Print and shaded views of the part. All mm, measured from the part's lowest x, y and z. A direction names the side the tool comes from. Round coordinates to 2 decimals unless told otherwise and drop trailing zeros. Order: outer loops, then holes, each group sorted by start corner. A loop starts at its lowest first (then second) coordinate and runs counter-clockwise, first axis right, second up. Notation, with made-up numbers: (-15.5, 61.25) -> (19.5, 61.25) arc R21 ccw to (19.5, 93.25) -> close; hole circle Ø5 at (3.25, 69). An arc over 180 degrees is marked (long way). Answer as CSV lines item,"result".
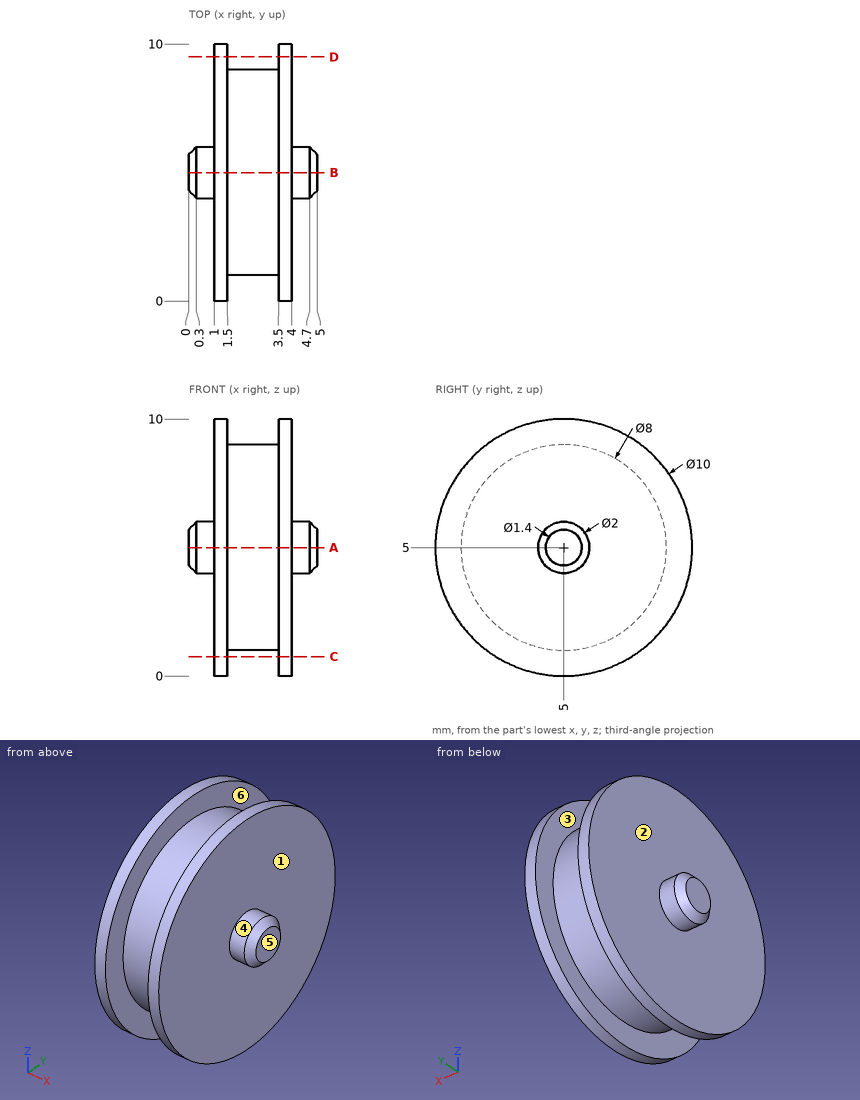
Q1. Saw through at A-A (z = 5). Write the cut outline in (x, y), plus the area to 3 significant figures.
Checks:
outline,"(0, 4.3) -> (0.3, 4) -> (1, 4) -> (1, 0) -> (1.5, 0) -> (1.5, 1) -> (3.5, 1) -> (3.5, 0) -> (4, 0) -> (4, 4) -> (4.7, 4) -> (5, 4.3) -> (5, 5.7) -> (4.7, 6) -> (4, 6) -> (4, 10) -> (3.5, 10) -> (3.5, 9) -> (1.5, 9) -> (1.5, 10) -> (1, 10) -> (1, 6) -> (0.3, 6) -> (0, 5.7) -> close"
area,"29.8 mm²"
Q2. Flat gauge pin, fed straight in: pin 1 (3 mm diameter, centred on y = 2.5, z = 5.5, fed in from +X). Where does the tip first touch, or does it go through?
Checks:
pin 1,"x = 4"
Q3. Saw through at D-D (y = 9.5). Write the cut outline in (x, z).
Checks:
outline,"(1, 2.82) -> (1.5, 2.82) -> (1.5, 7.18) -> (1, 7.18) -> close; (3.5, 2.82) -> (4, 2.82) -> (4, 7.18) -> (3.5, 7.18) -> close"
Q4. Mould opens along X. For the marked faces 1, 2, 3 and 4 say: +X half, -X half, draft (parallel to the pull), parting line (faces both ways), or undercut.
Checks:
face 1,"+X half"
face 2,"-X half"
face 3,"undercut"
face 4,"draft"
Q5. Tool access for the marked faces 5 and 6: list every direction of +Z, -Z, +X, -X, +Y, -Y with a clear straight run to the whole face (end or side of a thin tool).
Checks:
face 5,"+Z, -Z, +X, +Y, -Y"
face 6,"none"
Q6. Saw through at C-C (z = 0.75). Write the cut outline in (x, y).
Checks:
outline,"(1, 2.37) -> (1.5, 2.37) -> (1.5, 7.63) -> (1, 7.63) -> close; (3.5, 2.37) -> (4, 2.37) -> (4, 7.63) -> (3.5, 7.63) -> close"
Q7. Wall check: L1, parallel to X at y = 5.5, z = 8.25; L2, parallel to X at y = 6.25, z = 1; L3, parallel to Y at x = 4.65, z = 5. Give the ranges that are in metal, low to high. Write a range as [from, to].
Checks:
L1,"[1, 4]"
L2,"[1, 1.5], [3.5, 4]"
L3,"[4, 6]"
